For this review, use the dimensioned drawing (mm, ordinates from the lowest corner) and the shaded views. A direction names the side the tool comes from. Coordinates: 2 decimals unless noted, no trailing zeros. Order: outer loops, then holes, each group sorted by start corner. A loop starts at its lowest first (then second) coordinate and runs counter-clockwise, first axis right, second up. Notation, with made-up numbers: M 78.25,71.25 L 125.25,71.25 A16 ccw 125.25,98.25 Z; hole C -21,-17 d11. An arc over 180 degrees is marked long. One line per item, written item: value.
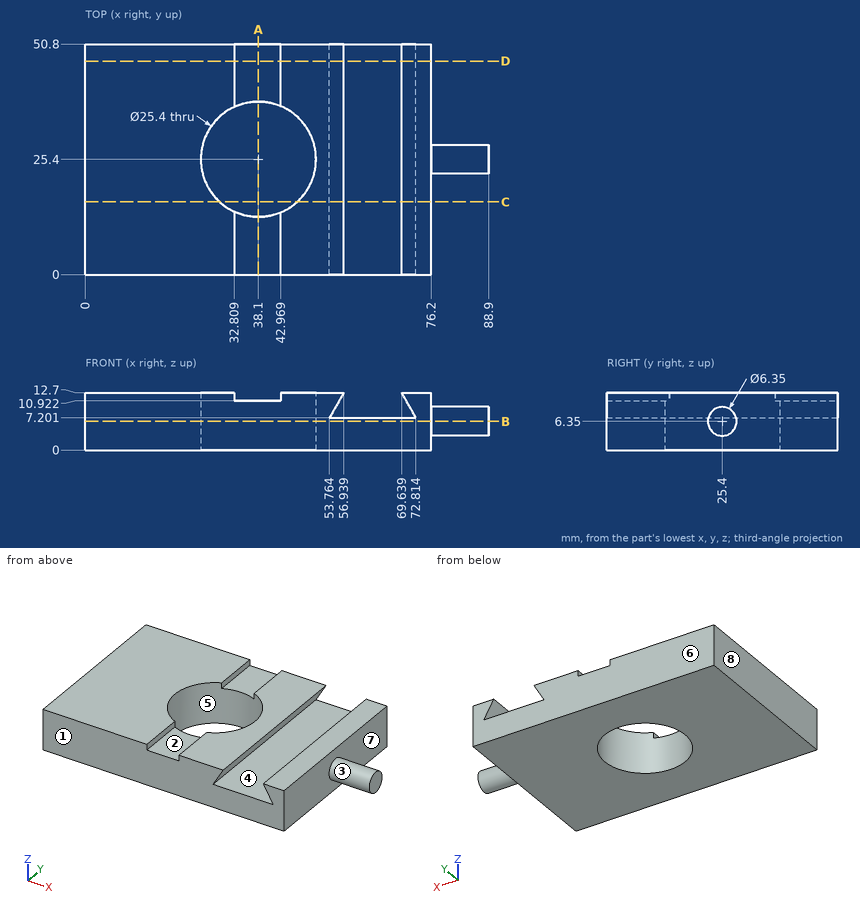
(1) For L1, parallel to Y at x = 38.1, z = 4.25; L2, parallel to X at y = 25, z = 2; L3, parallel to X at y = 25.4, z = 5.5, list the stretches that pass through material, from the lowest coordinate up.
Geometry results:
L1: y = 0 to 12.7, 38.1 to 50.8
L2: x = 0 to 25.41, 50.79 to 76.2
L3: x = 0 to 25.4, 50.8 to 88.9
(2) We need section C-C, the plane y = 16. State the section outline as (x, z) points.
Geometry results:
outline: M 0,0 L 29.56,0 L 29.56,12.7 L 0,12.7 Z; M 46.64,0 L 76.2,0 L 76.2,12.7 L 69.64,12.7 L 72.81,7.2 L 53.76,7.2 L 56.94,12.7 L 46.64,12.7 Z
(3) Insertion check: pin 1 Ø0.9 at (y, z) = (5, 11.5) entering from +X; pin 2 Ø3 at (x, y) = (39.5, 41) entering from +Z; pin 3 Ø1 at (x, y) = (59.5, 40) entering from +Z; pin 4 Ø6 at (x, y) = (35, 34.5) entering from +Z. Each pin has a flat end and moves straight along its axis. Give the tip position at first contact, or say it passes through.
Geometry results:
pin 1: stops at x = 76.2
pin 2: stops at z = 10.92
pin 3: stops at z = 7.2
pin 4: passes through
(4) We need section D-D, the plane y = 47. State the section outline as (x, z) points, plus the area to 3 significant figures.
Geometry results:
outline: M 0,0 L 76.2,0 L 76.2,12.7 L 69.64,12.7 L 72.81,7.2 L 53.76,7.2 L 56.94,12.7 L 42.97,12.7 L 42.97,10.92 L 32.81,10.92 L 32.81,12.7 L 0,12.7 Z
area: 862 mm2
(5) Mouldability with a two-part tool opening along X and no side actions: class the marked faces 5, 6, 7 and 8 as +X half, -X half, draft (parallel to the pull), parting line (faces both ways), or undercut.
Geometry results:
face 5: undercut
face 6: draft
face 7: +X half
face 8: -X half
(6) Tool access review of the marked faces 1, 2, 3 and 4: name each direction out of +Z, -Z, +X, -X, +Y, -Y from which nothing blocks a thin tool from reaching the whole face with its end or side.
Geometry results:
face 1: +Z, -Z, +X, -X, -Y
face 2: +Z, +Y, -Y
face 3: +X
face 4: +Y, -Y
(7) We need section A-A, the plane x = 38.1. State the section outline as (y, z) points, plus the area to 3 significant figures.
Geometry results:
outline: M 0,0 L 12.7,0 L 12.7,10.92 L 0,10.92 Z; M 38.1,0 L 50.8,0 L 50.8,10.92 L 38.1,10.92 Z
area: 277 mm2
(8) We need section B-B, the plane z = 6.35. State the section outline as (x, y) points (1 decimal), plus the area to 4 significant figures.
Geometry results:
outline: M 0,0 L 76.2,0 L 76.2,22.2 L 88.9,22.2 L 88.9,28.6 L 76.2,28.6 L 76.2,50.8 L 0,50.8 Z; hole C 38.1,25.4 d25.4
area: 3,445 mm2
